from build123d import *

# Parameters (mm, degrees)
CUT_EXTRUDE1_DEPTH      = 107.044923952
CUT_EXTRUDE1_DEPTH_BACK = 107.044923952
SKETCH2_R               = 1.651
CUT_EXTRUDE2_DEPTH      = 25.4
CHAMFER1_SIZE           = 0.762


with BuildPart() as part:
    # Sketch1 → Revolve1 (revolve)
    with BuildSketch(Plane.XY, mode=Mode.PRIVATE) as revolve1_sk:
        Polygon((0, 0), (0, 4.826), (-71.374, 4.826), (-71.374, 6.35), (-105.664, 6.35), (-105.664, 0), align=None)
    revolve(revolve1_sk.sketch.rotate(Axis((-91.219448406, 0, 0), (1, 0, 0)), 90), axis=Axis((-91.219448406, 0, 0), (1, 0, 0)))

    # Sketch2 → Cut-Extrude1 (cut, two sides: drawn at the far end of the back side and taken through both)
    with BuildSketch(Plane.XY.offset(-CUT_EXTRUDE1_DEPTH_BACK)):
        with Locations((-28.702, 0)):
            Circle(SKETCH2_R)
    extrude(amount=CUT_EXTRUDE1_DEPTH + CUT_EXTRUDE1_DEPTH_BACK, mode=Mode.SUBTRACT)

    # Sketch4 → Cut-Extrude2 (cut)
    with BuildSketch(Plane.ZY.offset(105.664)):
        with BuildLine():
            Line((-4.12701151, 4.826), (4.12701151, 4.826))
            ThreePointArc((4.12701151, 4.826), (0, 6.35), (-4.12701151, 4.826))
        make_face()
    extrude(amount=-CUT_EXTRUDE2_DEPTH, mode=Mode.SUBTRACT)

    # Chamfer1
    chamfer1_edges = [part.edges().sort_by_distance(p)[0] for p in [
        (-105.664, -5.76753947, -2.656687497),
    ]]
    chamfer(chamfer1_edges, length=CHAMFER1_SIZE)


solid = part.part
Check sheet for the modelled part. Datum: model origin and axes. Units: mm. A direction names the side the tool comes from. Round coordinates to 2 decimals unless told otherwise and drop trailing zeros. Loops run counter-clockwise (first coordinate to the right, second up) from the corner with the lowest first, then second, coordinate; pieces in that order, holes last.
1. Sectioned sample at A-A on y = 0. Record the boundary of the cut face in (x, z).
2. Scan lines: probe 1 along X at (y, z) = (0, 0.5); probe 2 along X at (y, z) = (0.25, 3); probe 3 along X at (y, z) = (2.25, -5). Record each from-to range of solid material in increasing order.
3. Sectioned sample at D-D on x = -97. Record the boundary of the cut face in (y, z).
4. Sectioned sample at B-B on z = 0. Record the boundary of the cut face in (x, y), and give its area (3 significant figures).
5. Sectioned sample at C-C on x = -42.5. Record the boundary of the cut face in (y, z).
6. Gauge pin test, flat ends, axial feed: pin 1 Ø1 at (x, y) = (-30, 1) entering from +Z; pin 2 Ø0.5 at (y, z) = (6, -1.5) entering from -X; pin 3 Ø3 at (x, z) = (-85, 4.5) entering from +Y; pin 4 Ø2 at (y, z) = (0, -3) entering from +X. Record the tip position at first contact, or that the pin passes through.
7. Set-up check for faces 5 (the cylindrical face through (-36.19, 4.71, -1.05)), 6 (the cylindrical face through (-88.4, -6.3, -0.8)): record each of +Z, -Z, +X, -X, +Y, -Y from which the full face is reachable in a straight line by a thin tool's end or side.
8. Mould release check, pull along Y, two halves, no side actions. Record for faces 1 (the flat face through (-71.374, -5, 1)), 2 (the conical face through (-105.54, -5.71, 0.21)), 3 (the flat face through (-93, 4.826, 0)), 4 (the cylindrical face through (-30.35, 0.07, -0.07)): released by +Y, released by -Y, zero draft, split by the parting line, or undercut.
Recorded:
1. outline: (-105.66, -5.59) - (-104.9, -6.35) - (-71.37, -6.35) - (-71.37, -4.83) - (-30.35, -4.83) - (-30.35, 4.83) - (-71.37, 4.83) - (-71.37, 6.35) - (-104.9, 6.35) - (-105.66, 5.59) - close; (-27.05, -4.83) - (0, -4.83) - (0, 4.83) - (-27.05, 4.83) - close
2. probe 1: x = -105.66 to -30.35, -27.05 to 0
2. probe 2: x = -105.66 to -30.33, -27.07 to 0
2. probe 3: x = -105.66 to -71.37
3. outline: (4.83, -4.13) - (4.83, 4.13) arc R6.35 ccw (long way) to start
4. outline: (-105.66, -5.59) - (-104.9, -6.35) - (-71.37, -6.35) - (-71.37, -4.83) - (0, -4.83) - (0, 4.83) - (-71.37, 4.83) - (-71.37, 6.35) - (-80.26, 6.35) - (-80.26, 4.83) - (-105.66, 4.83) - close; hole circle Ø3.3 at (-28.7, 0)
4. area: 1,080 mm2
5. outline: circle Ø9.65 at (0, 0)
6. pin 1: stops at z = 4.79
6. pin 2: stops at x = -80.26
6. pin 3: stops at y = 4.83
6. pin 4: stops at x = 0
7. face 5: +X
7. face 6: +X, -X
8. face 1: zero draft
8. face 2: split by the parting line
8. face 3: released by +Y
8. face 4: undercut
